Autodesk Inventor part; units mm, degrees
ref_plane "YZ Plane" through (0, 0, 0) normal (1, 0, 0) x (0, 1, 0)
ref_plane "XZ Plane" through (0, 0, 0) normal (0, 1, 0) x (-1, 0, 0)
ref_plane "XY Plane" through (0, 0, 0) normal (0, 0, 1) x (1, 0, 0)
sketch "スケッチ1" plane through (0, 0, 0) normal (0, 0, 1) x (1, 0, 0)
  arc A0 (0, 125) -> (-125, 0) centre (0, 0) ccw
  line L0 (0, 125) -> (0, 0)
  line L1 (0, 0) -> (-125, 0)
  point P0 (0, 0)
  dimension "d0" = 125
  dimension "d1" = 125
  dimension "d2" = 125
revolve "回転1" add sketch "スケッチ1" angle 360 about axis through (0, 125, 0) along (0, -1, 0)
sketch "スケッチ2" plane through (0, 0, 0) normal (0, -1, 0) x (1, 0, 0)
  line L0 (60, -130) -> (-60, -130)
  line L1 (-60, -130) -> (-60, 130)
  line L2 (-60, 130) -> (60, 130)
  line L3 (60, 130) -> (60, -130)
  line L4 (60, -130) -> (-60, 130) construction
  line L5 (-60, -130) -> (60, 130) construction
  line L6 (177.9877, -390) -> (60, -390)
  line L7 (60, -390) -> (60, 130)
  line L8 (60, 130) -> (177.9877, 130)
  line L9 (177.9877, 130) -> (177.9877, -390)
  line L10 (177.9877, -390) -> (60, 130) construction
  line L11 (60, -390) -> (177.9877, 130) construction
  point P0 (0, 0)
  point P1 (118.9938, -130)
  dimension "d4" = 120
  dimension "d5" = 260
extrude "押し出し1" cut sketch "スケッチ2" against normal blind 200
sketch "スケッチ3" plane through (0, 0, 0) normal (0, -1, 0) x (1, 0, 0)
  circle A0 centre (0, 0) radius 120
  line L0 (0, 0) -> (0, 7.6881)
  line L1 (0, 120) -> (0, -120)
  dimension "d8" = 240
revolve "回転2" cut sketch "スケッチ3" angle 360 about axis through (0, 0, 120) along (0, 0, -1) picked at (-69.9662, -38.4642) contours L1 L0 A0
properties material "PC/ABS プラスチック"
Check sheet for the modelled part. Datum: model origin and axes. Units: mm. Give positions to 0.01 mm unless a question says otherwise; leave off trailing zeros. Loops run counter-clockwise (first coordinate to the right, second up) from the corner with the lowest first, then second, coordinate; pieces in that order, holes last. Notation, with made-up numbers: M -12,-32 L 3,-32 A23 ccw 3,0 Z; hole C 63.5,24.5 d8. An arc over 180 degrees is marked long. Use a Markdown table: item, result. Add a question column.
Q1. Sectioned sample at B-B, the plane y = 83.5. Record the cut outline in (x, z), then the cut area to 3 significant figures.
Q2. Scan lines: line 1 along Z through (x, y) = (-93, 25.5); line 2 along Z through (x, y) = (-63, 14.5); line 3 along Y through (x, z) = (-104.5, 40). Record each from-to range of solid material in increasing order. Write a range as [from, to].
Q3. Sectioned sample at A-A, the plane z = -7.5. Record the cut outline in (x, y), then the cut area to 3 significant figures.
Q4. Go/stop test with flat-tipped pins: pin 1 (6 mm diameter, centred on x = -106, z = -0.5, fed in from +Y); pin 2 (3 mm diameter, centred on y = 59, z = 81, fed in from -X); pin 3 (1 mm diameter, centred on x = -76.5, z = -44, fed in from -Y). Record where each tip stops, or that it passes through.
Verdict:
| question | item | result |
|---|---|---|
| 1 | outline | M -60,-71.08 L -60,-61.87 A86.18 cw -60,61.87 L -60,71.08 A93.02 ccw Z |
| 1 | area | 1,030 mm^2 |
| 2 | line 1 | [-79.53, -71.42], [71.42, 79.53] |
| 2 | line 2 | [-106.98, -101.1], [101.1, 106.98] |
| 2 | line 3 | [43.36, 55.72] |
| 3 | outline | M -124.77,0 L -119.77,0 A119.77 cw -60,103.65 L -60,109.4 A124.77 ccw Z |
| 3 | area | 648 mm^2 |
| 4 | pin 1 | y = 70.82 |
| 4 | pin 2 | x = -76.69 |
| 4 | pin 3 | y = 80.77 |
